```python
from build123d import *

# Parameters (mm, degrees)
SKETCH1_R           = 7.5
SKETCH1_R_2         = 5
BOSS_EXTRUDE1_DEPTH = 5


with BuildPart() as part:
    # Sketch1 → Boss-Extrude1 (new, symmetric)
    with BuildSketch(Plane.XY):
        with BuildLine():
            Line((-75, -12.5), (75, -12.5))
            Line((75, -12.5), (125, -99.102540378))
            ThreePointArc((125, -99.102540378), (142.075317547, -103.677857926), (146.650635095, -86.602540378))
            Line((146.650635095, -86.602540378), (96.650635095, 0))
            ThreePointArc((96.650635095, 0), (87.5, 9.150635095), (75, 12.5))
            Line((75, 12.5), (-75, 12.5))
            ThreePointArc((-75, 12.5), (-87.5, 9.150635095), (-96.650635095, 0))
            Line((-96.650635095, 0), (-121.650635095, -43.301270189))
            ThreePointArc((-121.650635095, -43.301270189), (-117.075317547, -60.376587737), (-100, -55.801270189))
            Line((-100, -55.801270189), (-75, -12.5))
        make_face()
        Circle(SKETCH1_R, mode=Mode.SUBTRACT)
        with Locations((135.825317547, -92.852540378)):
            Circle(SKETCH1_R_2, mode=Mode.SUBTRACT)
        with Locations((-110.825317547, -49.551270189)):
            Circle(SKETCH1_R_2, mode=Mode.SUBTRACT)
    extrude(amount=BOSS_EXTRUDE1_DEPTH, both=True)


solid = part.part
```
Part model, mm, in its own coordinate system. A direction names the side the tool comes from. Coordinates: 2 decimals unless noted, no trailing zeros. Order: outer loops, then holes, each group sorted by start corner. A loop starts at its lowest first (then second) coordinate and runs counter-clockwise, first axis right, second up. Notation, with made-up numbers: (17, -26) -> (29, -26) arc R19 cw to (29, -21) -> close; hole circle Ø6 at (65, -1.75). An arc over 180 degrees is marked (long way). Put each result on its own line as item: value. Start each with the question number.
(1) Mould opens along Y. For faces 3 (the face through (131.857, -95.895, -0.07)), 4 (the face through (-7.493, 0.33, -0.07)), 5 (the face through (-1, -12.5, 0)), 6 (the face through (-117.312, -60.237, 0.07)) say: pulls with the +Y half, pulls with the -Y half, needs draft (parallel to the pull), parting line crosses it, or undercut.
(2) Which spindle directions (+Z, -Z, +X, -X, +Y, -Y) get a long thin tool onto all of the face, cutting with end or side? Do faces 1 (the face through (22, -11, -5)), 2 (the face through (99.65, -55.195, 0.07)). Say none if no direction does.
(3) Probe line 1 along X through (y, z) = (-53.5, -0.5); line 2 along Y through (x, z) = (0, -2.25); line 3 along Y through (x, z) = (-72.5, -1.25). List the from-to ranges inside material, lowest first. Write a range as [from, to].
(4) Band-saw the part on D-D (x = -60). Give the cut face in (y, z).
(5) Band-saw the part on C-C (y = -80.5). Give the cut face in (x, z).
(6) Pin check, flat tips, straight feed: pin 1 Ø4 at (y, z) = (-51, -1.5) entering from +X; pin 2 Ø5 at (x, z) = (-27, 1) entering from -Y; pin 3 Ø4 at (y, z) = (-39.5, -1) entering from -X. Stop position of each tip, or through.
(7) Band-saw the part on A-A (x = 0). Give the cut face in (y, z).
(8) Band-saw the part on B-B (z = 1). Give the cut face in (x, y), then the cut area to 3 significant figures.
Determined:
1. face 3: undercut
1. face 4: undercut
1. face 5: pulls with the -Y half
1. face 6: parting line crosses it
2. face 1: -Z, +X, -X, +Y, -Y
2. face 2: +Z, -Z, -Y
3. line 1: x = [-122.69, -113.89], [-107.76, -98.67], [98.67, 127.54]
3. line 2: y = [-12.5, -7.5], [7.5, 12.5]
3. line 3: y = [-12.5, 12.5]
4. outline: (-12.5, -5) -> (12.5, -5) -> (12.5, 5) -> (-12.5, 5) -> close
5. outline: (114.26, -5) -> (143.13, -5) -> (143.13, 5) -> (114.26, 5) -> close
6. pin 1: stops at x = 127.25
6. pin 2: stops at y = -12.5
6. pin 3: stops at x = -120.61
7. outline: (-12.5, -5) -> (-7.5, -5) -> (-7.5, 5) -> (-12.5, 5) -> close; (7.5, -5) -> (12.5, -5) -> (12.5, 5) -> (7.5, 5) -> close
8. outline: (-121.65, -43.3) arc R12.5 ccw to (-100, -55.8) -> (-75, -12.5) -> (75, -12.5) -> (125, -99.1) arc R12.5 ccw to (146.65, -86.6) -> (96.65, 0) arc R25 ccw to (75, 12.5) -> (-75, 12.5) arc R25 ccw to (-96.65, 0) -> close; hole circle Ø10 at (-110.83, -49.55); hole circle Ø15 at (0, 0); hole circle Ø10 at (135.83, -92.85)
8. area: 8,310 mm²
